Design review of the part shown in the three views and the two pictorial views. Dimensions are in mm from the part's minimum x, y and z. A direction names the side the tool comes from. Round coordinates to 2 decimals unless told otherwise and drop trailing zeros. Loops run counter-clockwise (first coordinate to the right, second up) from the corner with the lowest first, then second, coordinate; pieces in that order, holes last. Notation, with made-up numbers: (-24, -9) -> (-13, -9) arc R14 ccw to (-13, 18) -> close; hole circle Ø8 at (32.25, -19.5). An arc over 180 degrees is marked (long way). Return JSON: item names as keys, results as strings. Group by question number.
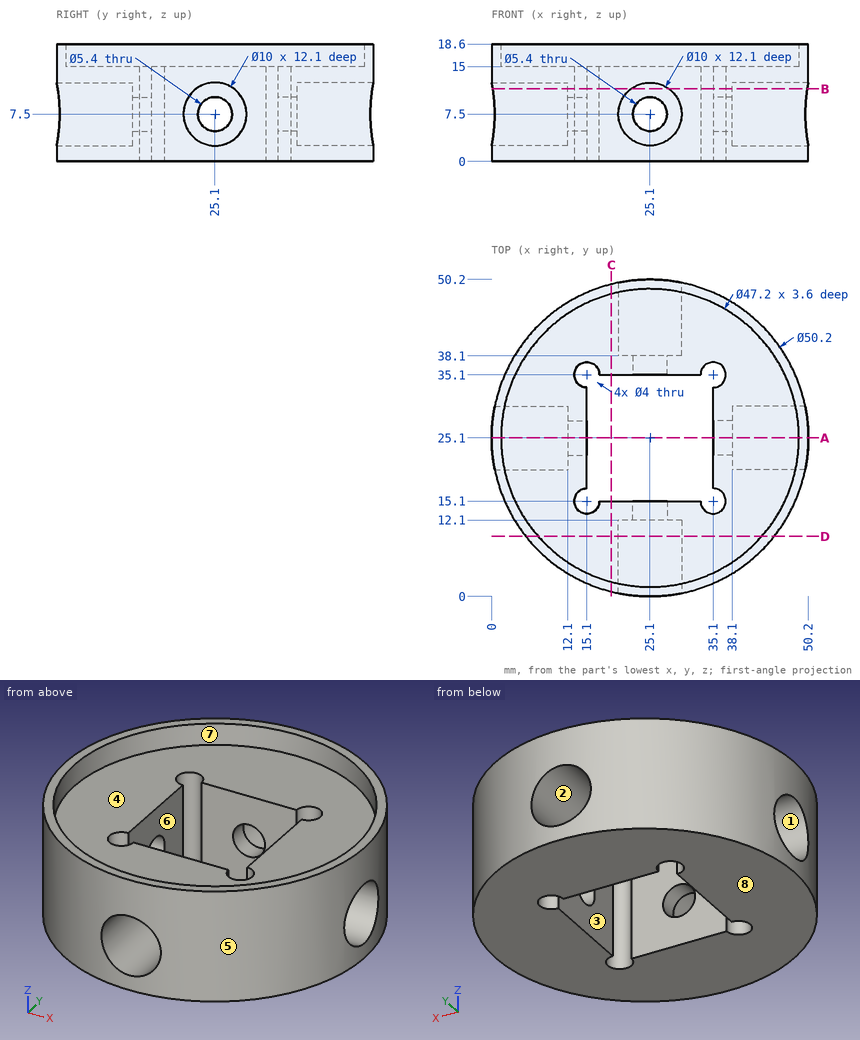
1. We need section B-B, the plane z = 11.5. Write out the cut boundary in (x, y).
2. Wall thickness on line 1 (Z direction, x = 25, y = 13); line 2 (Z direction, x = 33, y = 38.5); line 3 (Y direction, x = 32, z = 13.5): over which ranges is each line inside the solid? List them lowest first.
3. We need section A-A, the plane y = 25.1. Write out the cut boundary in (x, z), then the cut area to 3 significant figures.
4. Tool access review of the marked faces 1, 2, 3 and 4: name each direction out of +Z, -Z, +X, -X, +Y, -Y from which nothing blocks a thin tool from reaching the whole face with its end or side.
5. We need section C-C, the plane x = 19. Write out the cut boundary in (y, z), then the cut area to 3 significant figures.
6. For P1, Ø5, axis at x = 26.5, z = 7.5, coming from the -Y side; P2, Ø1, axis at x = 6, z = 14, coming from the +Y side; P3, Ø5, axis at x = 35.1, y = 35.1, coming from the +Z side; P4, Ø8, axis at x = 26, z = 9, coming from the +Y side, all flat-tipped, find the tip position at first contact; note any pin that passes through.
7. Draft analysis for pull direction Y (two halves, no side actions). For the marked faces 5, 6, 7 and 8, state which applies: pulls with the +Y half, pulls with the -Y half, needs draft (parallel to the pull), parting line crosses it, or undercut.
8. We need section D-D, the plane y = 9.5. Write out the cut boundary in (x, z).
Check sheet entries:
{
 "1": {"outline": "(0.18, 22.1) arc R25.1 ccw to (22.1, 0.18) -> (22.1, 12.1) -> (28.1, 12.1) -> (28.1, 0.18) arc R25.1 ccw to (50.02, 22.1) -> (38.1, 22.1) -> (38.1, 28.1) -> (50.02, 28.1) arc R25.1 ccw to (28.1, 50.02) -> (28.1, 38.1) -> (22.1, 38.1) -> (22.1, 50.02) arc R25.1 ccw to (0.18, 28.1) -> (12.1, 28.1) -> (12.1, 22.1) -> close; hole (15.1, 17.1) arc R2 ccw (long way) to (17.1, 15.1) -> (33.1, 15.1) arc R2 ccw (long way) to (35.1, 17.1) -> (35.1, 33.1) arc R2 ccw (long way) to (33.1, 35.1) -> (17.1, 35.1) arc R2 ccw (long way) to (15.1, 33.1) -> close"},
 "2": {"line 1": "z = 0 to 4.8, 10.2 to 15", "line 2": "z = 0 to 15", "line 3": "y = 0.97 to 15.1, 35.1 to 49.23"},
 "3": {"outline": "(0, 0) -> (15.1, 0) -> (15.1, 4.8) -> (12.1, 4.8) -> (12.1, 2.5) -> (0, 2.5) -> close; (0, 12.5) -> (12.1, 12.5) -> (12.1, 10.2) -> (15.1, 10.2) -> (15.1, 15) -> (1.5, 15) -> (1.5, 18.6) -> (0, 18.6) -> close; (35.1, 0) -> (50.2, 0) -> (50.2, 2.5) -> (38.1, 2.5) -> (38.1, 4.8) -> (35.1, 4.8) -> close; (35.1, 10.2) -> (38.1, 10.2) -> (38.1, 12.5) -> (50.2, 12.5) -> (50.2, 18.6) -> (48.7, 18.6) -> (48.7, 15) -> (35.1, 15) -> close", "area": "189 mm²"},
 "4": {"face 1": "-X", "face 2": "+Y", "face 3": "+Z, -Z", "face 4": "+Z"},
 "5": {"outline": "(0.75, 0) -> (15.1, 0) -> (15.1, 15) -> (2.3, 15) -> (2.3, 18.6) -> (0.75, 18.6) -> close; (35.1, 0) -> (49.45, 0) -> (49.45, 18.6) -> (47.9, 18.6) -> (47.9, 15) -> (35.1, 15) -> close", "area": "442 mm²"},
 "6": {"P1": "stops at y = 12.1", "P2": "stops at y = 41.95", "P3": "stops at z = 15", "P4": "stops at y = 50.2"},
 "7": {"face 5": "parting line crosses it", "face 6": "undercut", "face 7": "undercut", "face 8": "needs draft"},
 "8": {"outline": "(5.44, 0) -> (44.76, 0) -> (44.76, 18.6) -> (42.81, 18.6) -> (42.81, 15) -> (7.39, 15) -> (7.39, 18.6) -> (5.44, 18.6) -> close; hole circle Ø10 at (25.1, 7.5)"}
}
